from build123d import *

# Parameters (mm, degrees)
BOSS_EXTRU_1_DEPTH            = 12
ESQUISSE2_R                   = 1.55
ENL_V_MAT_EXTRU_1_DEPTH       = 16.94179588
ENL_V_START                   = -3
ESQUISSE3_R                   = 3
ENL_V_MAT_EXTRU_2_DEPTH       = 25
ENL_V_MAT_EXTRU_3_DEPTH       = 16.94179588
ENL_V_MAT_EXTRU_3_DEPTH_BACK  = 16.94179588
ESQUISSE4_R                   = 125
ENL_V_START_2                 = -12
ENL_V_MAT_EXTRU_4_DEPTH       = 1.613248654
ENL_V_START_3                 = 10.386751346
ENL_V_MAT_EXTRU_4_2_DEPTH     = 1.613248654
ENL_V_START_4                 = -4.63527657
ENL_V_MAT_EXTRU_4_3_OUTLINE_W = 24
ENL_V_MAT_EXTRU_4_3_OUTLINE_H = 5
ENL_V_MAT_EXTRU_4_3_DEPTH     = 2.892118763
ENL_V_START_5                 = -1.893983464
ENL_V_MAT_EXTRU_4_4_DEPTH     = 8.893983464
ENL_V_START_6                 = -7.5
ENL_V_MAT_EXTRU_4_5_DEPTH     = 15
CONG_1_R                      = 1


with BuildPart() as part:
    # Esquisse1 → Boss.-Extru.1 (new, symmetric)
    with BuildSketch(Plane(origin=(0, 0, 0), x_dir=(0, 0, -1), z_dir=(1, 0, 0))):
        Polygon((-3.863703305, 1.03527618), (4.829629131, -1.294095226), (4.829629131, 6.988114218), (-3.863703305, 9.317485624), align=None)
    extrude(amount=BOSS_EXTRU_1_DEPTH, both=True)

    # Esquisse2 → Enlèv. mat.-Extru.1 (cut, through all)
    with BuildSketch(Plane(origin=(0, 0, 0), x_dir=(1, 0, 0), z_dir=(0, -0.9659258262890672, 0.2588190451025247))):
        with Locations(Location((-8, 0, 0), (0, 0, 270))):
            Circle(ESQUISSE2_R)
        with Locations(Location((8, 0, 0), (0, 0, 270))):
            Circle(ESQUISSE2_R)
    extrude(amount=-ENL_V_MAT_EXTRU_1_DEPTH, mode=Mode.SUBTRACT)

    # Esquisse3 → Enlèv. mat.-Extru.2 (cut)
    with BuildSketch(Plane(origin=(0, 0, 0), x_dir=(1, 0, 0), z_dir=(0, -0.9659258262890672, 0.2588190451025247)).offset(ENL_V_START)):
        with Locations(Location((-8, 0, 0), (0, 0, 270))):
            Circle(ESQUISSE3_R)
        with Locations(Location((8, 0, 0), (0, 0, 270))):
            Circle(ESQUISSE3_R)
    extrude(amount=-ENL_V_MAT_EXTRU_2_DEPTH, mode=Mode.SUBTRACT)

    # Esquisse4 → Enlèv. mat.-Extru.3 (cut, two sides: drawn at the far end of the back side and taken through both)
    with BuildSketch(Plane(origin=(0, 0, 0), x_dir=(1, 0, 0), z_dir=(0, 1, 0)).offset(-ENL_V_MAT_EXTRU_3_DEPTH_BACK)):
        with Locations((0, 128.9)):
            Circle(ESQUISSE4_R)
    extrude(amount=ENL_V_MAT_EXTRU_3_DEPTH + ENL_V_MAT_EXTRU_3_DEPTH_BACK, mode=Mode.SUBTRACT)

    # Enlèv. mat.-Extru.4: read off the stored shape, not the designer's step
    # Enlèv. mat.-Extru.4 outline → Enlèv. mat.-Extru.4 (cut)
    with BuildSketch(Plane.YZ.offset(ENL_V_START_2)):
        Polygon((9.317485624, 3.863703305), (4.141104722, 3.863703305), (2.44661504, -2.46021828), (8.023390398, -0.965925826), align=None)
    extrude(amount=ENL_V_MAT_EXTRU_4_DEPTH, mode=Mode.SUBTRACT)

    # Enl_v. mat.-Extru.4 2 outline → Enl_v. mat.-Extru.4 2 (cut)
    with BuildSketch(Plane.YZ.offset(ENL_V_START_3)):
        Polygon((9.317485624, 3.863703305), (4.141104722, 3.863703305), (2.44661504, -2.46021828), (8.023390398, -0.965925826), align=None)
    extrude(amount=ENL_V_MAT_EXTRU_4_2_DEPTH, mode=Mode.SUBTRACT)

    # Enl_v. mat.-Extru.4 3 outline → Enl_v. mat.-Extru.4 3 (cut)
    with BuildSketch(Plane(origin=(0, 0, 0), x_dir=(1, 0, 0), z_dir=(0, 0.25881904510252507, 0.9659258262890671)).offset(ENL_V_START_4)):
        with Locations((0, 5.5)):
            Rectangle(ENL_V_MAT_EXTRU_4_3_OUTLINE_W, ENL_V_MAT_EXTRU_4_3_OUTLINE_H)
    extrude(amount=ENL_V_MAT_EXTRU_4_3_DEPTH, mode=Mode.SUBTRACT)

    # Enl_v. mat.-Extru.4 4 outline → Enl_v. mat.-Extru.4 4 (cut)
    with BuildSketch(Plane(origin=(0, 0, 0), x_dir=(1, 0, 0), z_dir=(0, 0.25881904510252507, 0.9659258262890671)).offset(ENL_V_START_5)):
        Polygon((-12, 8), (-12, 3), (-10.386751346, 3), (-7.5, 8), align=None)
        Polygon((12, 8), (7.5, 8), (10.386751346, 3), (12, 3), align=None)
    extrude(amount=ENL_V_MAT_EXTRU_4_4_DEPTH, mode=Mode.SUBTRACT)

    # Enl_v. mat.-Extru.4 5 outline → Enl_v. mat.-Extru.4 5 (cut)
    with BuildSketch(Plane.YZ.offset(ENL_V_START_6)):
        Polygon((7.276244171, -3.754313506), (8.023390398, -0.965925826), (2.44661504, -2.46021828), align=None)
    extrude(amount=ENL_V_MAT_EXTRU_4_5_DEPTH, mode=Mode.SUBTRACT)

    # Congé1
    # the kernel refuses this fillet: 1 mm, written as the material it adds along each edge
    with BuildSketch(Plane(origin=(-10.386751346, 4.514677836, 5.257897145), x_dir=(-1, 0, 0), z_dir=(0, -0.2588190451454881, -0.9659258262775553))) as cong_1_piece_1_section:
        with BuildLine():
            CenterArc((CONG_1_R * 0.577350268999, CONG_1_R), CONG_1_R, 210, 60)
            Line((-CONG_1_R * 0.288675134782, CONG_1_R * 0.499999999993), (0, 0))
            Line((0, 0), (CONG_1_R * 0.577350268999, 0))
        make_face()
    cong_1_piece_1 = extrude(amount=5.873068178, mode=Mode.PRIVATE)
    cong_1_piece_1 = split(cong_1_piece_1, bisect_by=Plane(origin=(-10.386751346, 4.514677836, 3.863703305), z_dir=(0, 0, -1)), keep=Keep.TOP, mode=Mode.PRIVATE)
    cong_1_piece_1 = cong_1_piece_1 - Plane(origin=(-8, 2.897777479, -0.776457135), x_dir=(0, -0.25881904510252474, -0.9659258262890673), z_dir=(0, -0.9659258262890673, 0.25881904510252474)) * Cylinder(3, 15, mode=Mode.PRIVATE)
    add(cong_1_piece_1)
    with BuildSketch(Plane(origin=(-7.00177766, 2.44661504, -2.46021828), x_dir=(0, -0.2588190451025249, -0.9659258262890672), z_dir=(1, 0, 0))) as cong_1_piece_2_section:
        with BuildLine():
            CenterArc((CONG_1_R * 0.577350268769, CONG_1_R), CONG_1_R, 210.000000004, 59.999999996)
            Line((-CONG_1_R * 0.288675134977, CONG_1_R * 0.499999999934), (0, 0))
            Line((0, 0), (CONG_1_R * 0.577350268769, 0))
        make_face()
    cong_1_piece_2 = extrude(amount=14.003555319, mode=Mode.PRIVATE)
    cong_1_piece_2 = cong_1_piece_2 - Plane(origin=(-8, 2.897777479, -0.776457135), x_dir=(0, -0.25881904510252474, -0.9659258262890673), z_dir=(0, -0.9659258262890673, 0.25881904510252474)) * Cylinder(3, 31, mode=Mode.PRIVATE)
    cong_1_piece_2 = cong_1_piece_2 - Plane(origin=(8, 2.897777479, -0.776457135), x_dir=(0, -0.25881904510252474, -0.9659258262890673), z_dir=(0, -0.9659258262890673, 0.25881904510252474)) * Cylinder(3, 31, mode=Mode.PRIVATE)
    add(cong_1_piece_2)
    with BuildSketch(Plane(origin=(10.386751346, 4.514677836, 5.257897145), x_dir=(-0.5000000002478059, 0.8365163035896415, -0.22414386804219472), z_dir=(0, -0.2588190451454881, -0.9659258262775553))) as cong_1_piece_3_section:
        with BuildLine():
            CenterArc((CONG_1_R * 0.577350268999, CONG_1_R), CONG_1_R, 210.000000016, 60)
            Line((-CONG_1_R * 0.288675134643, CONG_1_R * 0.499999999752), (0, 0))
            Line((0, 0), (CONG_1_R * 0.577350269277, 0))
        make_face()
    cong_1_piece_3 = extrude(amount=5.873068178, mode=Mode.PRIVATE)
    cong_1_piece_3 = split(cong_1_piece_3, bisect_by=Plane(origin=(10.386751346, 4.514677836, 3.863703305), z_dir=(0, 0, -1)), keep=Keep.TOP, mode=Mode.PRIVATE)
    cong_1_piece_3 = cong_1_piece_3 - Plane(origin=(8, 2.897777479, -0.776457135), x_dir=(0, -0.25881904510252474, -0.9659258262890673), z_dir=(0, -0.9659258262890673, 0.25881904510252474)) * Cylinder(3, 15, mode=Mode.PRIVATE)
    add(cong_1_piece_3)
    # the kernel refuses this fillet: 1 mm, written as the material it takes off along each edge
    with BuildSketch(Plane(origin=(12, 6.641104722, 3.863703305), x_dir=(0, 0, -1), z_dir=(0, -1, 0))) as cong_1_2_piece_1:
        with BuildLine():
            CenterArc((CONG_1_R, -CONG_1_R), CONG_1_R, 90, 90)
            Line((0, -CONG_1_R), (0, 0))
            Line((0, 0), (CONG_1_R, 0))
        make_face()
    extrude(amount=8.105828542, mode=Mode.SUBTRACT)
    with BuildSketch(Plane(origin=(-12, 6.641104722, 3.863703305), x_dir=(0, 0, -1), z_dir=(0, -1, 0))) as cong_1_2_piece_2:
        with BuildLine():
            CenterArc((CONG_1_R, CONG_1_R), CONG_1_R, 180, 90)
            Line((0, CONG_1_R), (0, 0))
            Line((0, 0), (CONG_1_R, 0))
        make_face()
    extrude(amount=8.105828542, mode=Mode.SUBTRACT)
    with BuildSketch(Plane(origin=(-12, -3.940338157, -4.477333255), x_dir=(0, 0, 1), z_dir=(0, 1, 0))) as cong_1_2_piece_3:
        with BuildLine():
            CenterArc((1.096256131, 1), CONG_1_R, 174.991611749, 95.008388251)
            ThreePointArc((0.100074203, 1.087301587), (0.051224329, 0.543541522), (0, 0))
            Line((0, 0), (1.096256131, 0))
        make_face()
    extrude(amount=8.587109196, mode=Mode.SUBTRACT)
    with BuildSketch(Plane(origin=(12, -3.940338157, -4.477333255), x_dir=(-0.9957911285935623, 0, 0.09165166782093803), z_dir=(0, 1, 0))) as cong_1_2_piece_4:
        with BuildLine():
            CenterArc((1.096264831, 0.999990462), CONG_1_R, 174.741366539, 95.008388251)
            Line((0.100473703, 1.09164213), (0, 0))
            ThreePointArc((0, 0), (0.545948621, 0.001192245), (1.091897242, 0))
        make_face()
    extrude(amount=8.587109196, mode=Mode.SUBTRACT)


solid = part.part
Here's how the part is built. I have some questions about the finished solid (model axes, mm). Coordinates: 2 decimals unless noted, no trailing zeros. Write each loop counter-clockwise with the first axis right and the second up, starting at its lowest first coordinate (ties: lowest second). Pieces come first, ordered by that corner, then holes.
Item 1: If we mould it in two halves opening along Z, with no side actions, what happens to faces 1 (the cylindrical face through (6.625, 1.243, -1.074)), 2 (the flat face through (12, 2, 0)), 3 (the cylindrical face through (-0.2, 0.4, -3.9))? For each: +Z half, -Z half, draft (parallel to the pull), parting line (faces both ways), or undercut.
Item 2: I want a section at A-A on x = 8.75. Write out the boundary of the cut face in (y, z).
Item 3: I want a section at B-B on x = 1.5. Write out the boundary of the cut face in (y, z), and give its area (3 significant figures).
Item 4: If I drill on line 1 (Z direction, x = -7.25, y = 1.25); line 2 (Y direction, x = 8, z = -2.5); line 3 (X direction, y = 5, z = 3.75), over which ranges is the centre line in solid material (lowest first)?
Item 5: I want a section at C-C on z = 0.25. Count the separate pieces of the cut face and the enclosed holes in it, and give its area (3 significant figures).
Item 6: Will these pins go through, and if not, where does the flat tip stop? pin 1 (1 mm diameter, centred on x = -8, z = -1.5, fed in from -Y); pin 2 (1 mm diameter, centred on y = 7.5, z = 2, fed in from +X); pin 3 (3 mm diameter, centred on y = 5, z = 2.5, fed in from -X).
Item 7: I want a section at D-D on x = -9.25. Write out the boundary of the cut face in (y, z), and give its area (3 significant figures).
Findings below:
1. face 1: undercut
1. face 2: draft
1. face 3: -Z half
2. outline: (-1.13, -4.21) - (1.98, -4.21) - (2.55, -2.09) - (-0.35, -1.31) - close; (0.35, 1.31) - (3.25, 0.53) - (3.65, 2.03) - (6.39, 1.3) - (7.08, 3.86) - (1.04, 3.86) - close
3. outline: (-1.05, -3.91) - (2.06, -3.91) - (2.3, -3.02) arc R1 cw to (3, -2.31) - (8.02, -0.97) - (9.32, 3.86) - (1.04, 3.86) - close
3. area: 53.1 mm2
4. line 1: z = -4.11 to -1.74, 1.07 to 3.86
4. line 2: y = -0.67 to 2.44
4. line 3: x = -9.89 to 9.89
5. separate pieces: 3
5. enclosed holes: 0
5. area: 115 mm2
6. pin 1: stops at y = -0.54
6. pin 2: stops at x = 8.52
6. pin 3: stops at x = -12
7. outline: (-1.14, -4.24) - (1.97, -4.24) - (2.66, -1.66) - (-0.24, -0.89) - close; (0.24, 0.89) - (3.13, 0.11) - (3.6, 1.86) - (5.51, 1.35) - (6.18, 3.86) - (1.04, 3.86) - close
7. area: 24.3 mm2
